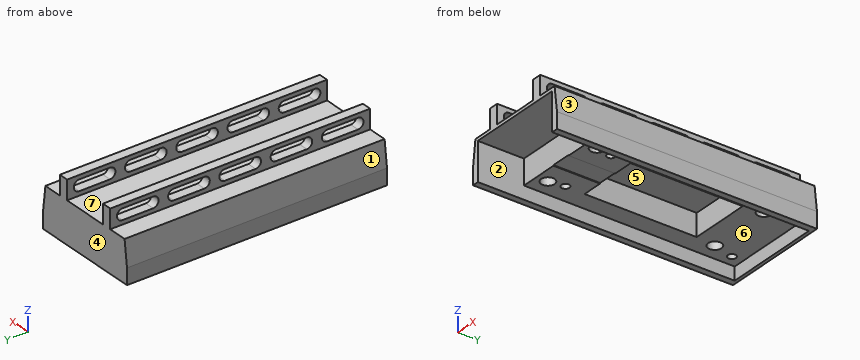
```python
from build123d import *

# Parameters (mm, degrees)
BOSS_EXTRUDE1_DEPTH             = 80.2
BOSS_EXTRUDE2_DEPTH             = 1
SKETCH4_W                       = 3
SKETCH4_H                       = 81.2
BOSS_EXTRUDE3_DEPTH             = 6
M3_START                        = 5.925
M3_CLEARANCE_SLOT1_DEPTH        = 20.8
SKETCH24_W                      = 20.25
SKETCH24_H                      = 3
CUT_EXTRUDE5_DEPTH              = 1
BOSS_EXTRUDE7_DEPTH             = 7.8
SKETCH31_W                      = 34.65
SKETCH31_H                      = 3
CUT_EXTRUDE6_DEPTH              = 95
SKETCH34_W                      = 6.25
SKETCH34_H                      = 14.559328602
BOSS_EXTRUDE8_DEPTH             = 7.6
SKETCH35_R                      = 2.1
CUT_EXTRUDE7_DEPTH              = 4
SKETCH36_W                      = 19
SKETCH36_H                      = 35
BOSS_EXTRUDE9_DEPTH             = 0.8
TAP_DRILL_FOR_M3X0_5_TAP1_D     = 2.5
TAP_DRILL_FOR_M3X0_5_TAP1_DEPTH = 6.5
TAP_DRILL_FOR_M3X0_5_TAP1_TIP   = 0.751075774
TAP_DRILL_FOR_M3X0_5_TAP2_D     = 2.5
TAP_DRILL_FOR_M3X0_5_TAP2_DEPTH = 6.5
TAP_DRILL_FOR_M3X0_5_TAP2_TIP   = 0.751075774


# Read off the part's stored shape, not the designer's step: M3 Clearance Slot1
with BuildPart() as part:
    # Sketch1 → Boss-Extrude1 (new body)
    with BuildSketch(Plane(origin=(0, 0, 0), x_dir=(1, 0, 0), z_dir=(0, 1, 0))):
        Polygon((0, 0), (32.65, 0), (33.65, 7.9), (33.65, 15.9), (31.65, 15.9), (31.65, 1), (1, 1), (1, 15.9), (-1, 15.9), (-1, 7.9), align=None)
    extrude(amount=BOSS_EXTRUDE1_DEPTH)

    # Sketch2 → Boss-Extrude2 (add)
    with BuildSketch(Plane(origin=(0, 80.2, 0), x_dir=(1, 0, 0), z_dir=(0, 1, 0))):
        Polygon((32.65, 0), (0, 0), (-1, 7.9), (-1, 15.9), (33.65, 15.9), (33.65, 7.9), align=None)
    extrude(amount=BOSS_EXTRUDE2_DEPTH)

    # Sketch4 → Boss-Extrude3 (add)
    with BuildSketch(Plane.XY):
        with Locations((25.225, 40.6)):
            Rectangle(SKETCH4_W, SKETCH4_H)
        with Locations((7.425, 40.6)):
            Rectangle(SKETCH4_W, SKETCH4_H)
    extrude(amount=BOSS_EXTRUDE3_DEPTH)

    # M3 Clearance Slot1 outline → M3 Clearance Slot1 (cut)
    with BuildSketch(Plane.YZ.offset(M3_START)):
        with BuildLine():
            ThreePointArc((13.4, 1.3), (15.1, 3), (13.4, 4.7))
            Line((13.4, 4.7), (3.8, 4.7))
            ThreePointArc((3.8, 4.7), (2.1, 3), (3.8, 1.3))
            Line((3.8, 1.3), (13.4, 1.3))
        make_face()
        with BuildLine():
            ThreePointArc((19.8, 4.7), (18.1, 3), (19.8, 1.3))
            Line((19.8, 1.3), (29.4, 1.3))
            ThreePointArc((29.4, 1.3), (31.1, 3), (29.4, 4.7))
            Line((29.4, 4.7), (19.8, 4.7))
        make_face()
        with BuildLine():
            ThreePointArc((35.8, 4.7), (34.1, 3), (35.8, 1.3))
            Line((35.8, 1.3), (45.4, 1.3))
            ThreePointArc((45.4, 1.3), (47.1, 3), (45.4, 4.7))
            Line((45.4, 4.7), (35.8, 4.7))
        make_face()
        with BuildLine():
            ThreePointArc((51.8, 4.7), (50.1, 3), (51.8, 1.3))
            Line((51.8, 1.3), (61.4, 1.3))
            ThreePointArc((61.4, 1.3), (63.1, 3), (61.4, 4.7))
            Line((61.4, 4.7), (51.8, 4.7))
        make_face()
        with BuildLine():
            ThreePointArc((67.8, 4.7), (66.1, 3), (67.8, 1.3))
            Line((67.8, 1.3), (77.4, 1.3))
            ThreePointArc((77.4, 1.3), (79.1, 3), (77.4, 4.7))
            Line((77.4, 4.7), (67.8, 4.7))
        make_face()
    extrude(amount=M3_CLEARANCE_SLOT1_DEPTH, mode=Mode.SUBTRACT)

    # Sketch24 → Cut-Extrude5 (cut)
    with BuildSketch(Plane(origin=(0, 81.2, 0), x_dir=(1, 0, 0), z_dir=(0, 1, 0))):
        with Locations((16.325, 14.4)):
            Rectangle(SKETCH24_W, SKETCH24_H)
    extrude(amount=-CUT_EXTRUDE5_DEPTH, mode=Mode.SUBTRACT)

    # Sketch30 → Boss-Extrude7 (add)
    with BuildSketch(Plane(origin=(0, 0, -1), x_dir=(-1, 0, 0), z_dir=(0, 0, -1))):
        Polygon((-26.8, 27.95), (-19.425, 27.95), (-19.425, 28.95), (-25.8, 28.95), (-25.8, 63.95), (-6.8, 63.95), (-6.8, 28.95), (-13.175, 28.95), (-13.175, 27.95), (-5.8, 27.95), (-5.8, 64.95), (-26.8, 64.95), align=None)
        Polygon((-31.65, 80.2), (-31.65, 27.95), (-26.8, 27.95), (-26.8, 64.95), (-5.8, 64.95), (-5.8, 27.95), (-1, 27.95), (-1, 80.2), align=None)
        Polygon((-31.65, 27.95), (-31.65, 14.390671398), (-19.425, 14.390671398), (-19.425, 27.95), (-26.8, 27.95), align=None)
        Polygon((-13.175, 27.95), (-13.175, 14.390671398), (-1, 14.390671398), (-1, 27.95), (-5.8, 27.95), align=None)
    extrude(amount=BOSS_EXTRUDE7_DEPTH)

    # Sketch31 → Cut-Extrude6 (cut)
    with BuildSketch(Plane.XZ):
        with Locations((16.325, -14.4)):
            Rectangle(SKETCH31_W, SKETCH31_H)
    extrude(amount=-CUT_EXTRUDE6_DEPTH, mode=Mode.SUBTRACT)

    # Sketch34 → Boss-Extrude8 (add)
    with BuildSketch(Plane(origin=(0, 0, -1), x_dir=(-1, 0, 0), z_dir=(0, 0, -1))):
        with Locations((-16.3, 21.670335699)):
            Rectangle(SKETCH34_W, SKETCH34_H)
    extrude(amount=BOSS_EXTRUDE8_DEPTH)

    # Sketch35 → Cut-Extrude7 (cut)
    with BuildSketch(Plane(origin=(0, 0, -8.8), x_dir=(-1, 0, 0), z_dir=(0, 0, -1))):
        with Locations((-26.475, 70.1)):
            Circle(SKETCH35_R)
        with Locations((-6.175, 70.1)):
            Circle(SKETCH35_R)
        with Locations((-6.175, 17.95)):
            Circle(SKETCH35_R)
        with Locations((-26.475, 17.95)):
            Circle(SKETCH35_R)
    extrude(amount=-CUT_EXTRUDE7_DEPTH, mode=Mode.SUBTRACT)

    # Sketch36 → Boss-Extrude9 (add)
    with BuildSketch(Plane(origin=(0, 0, -1), x_dir=(-1, 0, 0), z_dir=(0, 0, -1))):
        with Locations((-16.3, 46.45)):
            Rectangle(SKETCH36_W, SKETCH36_H)
    extrude(amount=BOSS_EXTRUDE9_DEPTH)

    # Tap Drill for M3x0.5 Tap1
    with Locations(Plane(origin=(28.15, 76.7, -8.8), x_dir=(-1, 0, 0), z_dir=(0, 0, -1))):
        with Locations((0, 0), (23.65, 0)):
            Hole(TAP_DRILL_FOR_M3X0_5_TAP1_D / 2, depth=TAP_DRILL_FOR_M3X0_5_TAP1_DEPTH)
            with Locations((0, 0, -(TAP_DRILL_FOR_M3X0_5_TAP1_DEPTH + TAP_DRILL_FOR_M3X0_5_TAP1_TIP / 2))):  # 118° drill point
                Cone(0, TAP_DRILL_FOR_M3X0_5_TAP1_D / 2, TAP_DRILL_FOR_M3X0_5_TAP1_TIP, mode=Mode.SUBTRACT)

    # Tap Drill for M3x0.5 Tap2
    with Locations(Plane(origin=(25.725, 22.85, -8.8), x_dir=(-1, 0, 0), z_dir=(0, 0, -1))):
        with Locations((0, 0), (18.8, 0)):
            Hole(TAP_DRILL_FOR_M3X0_5_TAP2_D / 2, depth=TAP_DRILL_FOR_M3X0_5_TAP2_DEPTH)
            with Locations((0, 0, -(TAP_DRILL_FOR_M3X0_5_TAP2_DEPTH + TAP_DRILL_FOR_M3X0_5_TAP2_TIP / 2))):  # 118° drill point
                Cone(0, TAP_DRILL_FOR_M3X0_5_TAP2_D / 2, TAP_DRILL_FOR_M3X0_5_TAP2_TIP, mode=Mode.SUBTRACT)


solid = part.part
```
Model file for the job. Use its own axes, mm. Face numbers are marked on the shaded views. A direction names the side the tool comes from. Give positions to 0.01 mm unless a question says otherwise; leave off trailing zeros. Order: outer loops, then holes, each group sorted by start corner. A loop starts at its lowest first (then second) coordinate and runs counter-clockwise, first axis right, second up.
1) Saw through at D-D, the plane y = 67. Write the cut outline in (x, z) (3 decimals), then the cut area to 3 significant figures.
2) Saw through at B-B, the plane x = 14. Write the cut outline in (y, z), then the cut area to 4 significant figures.
3) Pin check, flat tips, straight feed: pin 1 (12 mm diameter, centred on x = 14, y = 30, fed in from -Z); pin 2 (4 mm diameter, centred on x = 6.175, y = 70.1, fed in from -Z); pin 3 (4 mm diameter, centred on x = 2.5, y = 51, fed in from +Z). Stop position of each tip, or through.
4) Wall check: probe 1 along Z at (x, y) = (8, 11.5); probe 2 along X at (y, z) = (24, -12); probe 3 along Y at (x, z) = (28.15, -4.75). Give the ranges that are in metal, low to high.
5) Mould opens along X. For the marked faces 1, 2, 3 and 4 say: +X half, -X half, draft (parallel to the pull), parting line (faces both ways), or undercut.
6) 3-axis set-ups, long thin cutter, end or side, ignore diameter. For the marked faces 5, 6 and 7: which of +Z, -Z, +X, -X, +Y, -Y reach the whole face in a straight line?
7) Saw through at A-A, the plane y = 39. Count the separate pieces of the cut face and the enclosed holes in it, then the cut area to 3 significant figures.
Computed:
1. outline: (-1, -12.9) - (1, -12.9) - (1, -8.8) - (31.65, -8.8) - (31.65, -12.9) - (33.65, -12.9) - (33.65, -7.9) - (32.65, 0) - (26.725, 0) - (26.725, 1.5) - (23.725, 1.5) - (23.725, 0) - (8.925, 0) - (8.925, 1.5) - (5.925, 1.5) - (5.925, 0) - (0, 0) - (-1, -7.9) - close; (5.925, 4.5) - (8.925, 4.5) - (8.925, 6) - (5.925, 6) - close; (23.725, 4.5) - (26.725, 4.5) - (26.725, 6) - (23.725, 6) - close
1. area: 331 mm2
2. outline: (0, -1) - (14.39, -1) - (14.39, -8.6) - (28.95, -8.6) - (28.95, -1.8) - (63.95, -1.8) - (63.95, -8.8) - (80.2, -8.8) - (80.2, -12.9) - (81.2, -12.9) - (81.2, 0) - (0, 0) - close
2. area: 358.5 mm2
3. pin 1: stops at z = -8.8
3. pin 2: stops at z = -4.8
3. pin 3: stops at z = 0
4. probe 1: z = -1 to 1.3, 4.7 to 6
4. probe 2: x = -1 to 1, 31.65 to 33.65
4. probe 3: y = 14.39 to 75.45, 77.95 to 81.2
5. face 1: -X half
5. face 2: undercut
5. face 3: +X half
5. face 4: draft
6. face 5: -Z
6. face 6: -Z, -Y
6. face 7: +Z, +Y, -Y
7. separate pieces: 3
7. enclosed holes: 0
7. area: 196 mm2
